Could you check a few things on this model? Use its own coordinates, in mm. Coordinates: 2 decimals unless noted, no trailing zeros. Loops run counter-clockwise (first coordinate to the right, second up) from the corner with the lowest first, then second, coordinate; pieces in that order, holes last. Notation, with made-up numbers: M 1.25,45 L 21.25,45 A7 ccw 21.25,51 Z; hole C 56.25,54.25 d3. An arc over 180 degrees is marked long. Return JSON: item names as keys, results as strings. Group by question number.
from build123d import *

# Parameters (mm, degrees)
F1_DEPTH = 875


with BuildPart() as f1:
    # F0 (on Right) → F1 (new body)
    with BuildSketch(Plane.YZ):
        with BuildLine():
            Line((35, 150), (10.037331, 150))
            ThreePointArc((10.037331, 150), (0.000372, 146.147172), (-4.880497, 136.567927))
            Line((-4.880497, 136.567927), (-33.258641, -133.432073))
            ThreePointArc((-33.258641, -133.432073), (-29.487985, -145.036959), (-18.340812, -150))
            Line((-18.340812, -150), (35, -150))
            Line((35, -150), (35, 150))
        make_face()
    extrude(amount=F1_DEPTH)


solid = f1.part
(1) Imagine slicing it at C-C, the plane z = 19. Write out the boundary of the cut face in (x, y), then the cut area to 3 significant figures.
(2) Imagine slicing it at B-B, the plane z = -53.5. Write out the boundary of the cut face in (x, y), then the cut area to 3 significant figures.
(3) If I drill on L1, parallel to Z at x = 445, y = 9; L2, parallel to Y at x = 670, z = -136.5; L3, parallel to Y at x = 664.5, z = -55.5, over which ranges is the centre line in solid material (lowest first)? Write a range as [from, to].
(4) Imagine slicing it at A-A, the plane x = 507.5. Write out the boundary of the cut face in (y, z), then the cut area to 3 significant figures.
(5) Will these pins go through, and if not, where does the flat tip stop? P1, Ø6, axis at x = 351.5, z = 91.5, coming from the -Y side; P2, Ø3, axis at x = 644.5, z = -85.5, coming from the -Y side.
Checks:
{
 "1": {"outline": "M 0,-17.24 L 875,-17.24 L 875,35 L 0,35 Z", "area": "45,700 mm²"},
 "2": {"outline": "M 0,-24.86 L 875,-24.86 L 875,35 L 0,35 Z", "area": "52,400 mm²"},
 "3": {"L1": "[-150, 149.96]", "L2": "[-33.27, 35]", "L3": "[-25.07, 35]"},
 "4": {"outline": "M -33.26,-133.43 A15 ccw -18.34,-150 L 35,-150 L 35,150 L 10.04,150 A15 ccw -4.88,136.57 Z", "area": "16,200 mm²"},
 "5": {"P1": "y = -9.93", "P2": "y = -28.38"}
}
